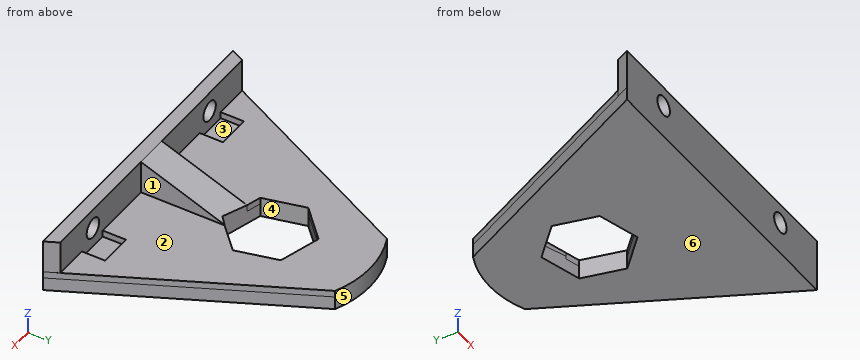
```python
from build123d import *

# Parameters (mm, degrees)
SKETCH_1_R               = 3
EXTRUDE_1_DEPTH          = 2
EXTRUDE_2_DEPTH          = 6
RIB_2_REACH              = 42.702
SKETCH_3_WALL_W          = 109.004825052
SKETCH_3_WALL_H          = 5
SKETCH_4_R               = 4.101413307
EXTRUDE_3_DEPTH          = 2
EXTRUDE_START            = -3
EXTRUDE_4_DEPTH          = 1
CUT_EXTRUDE_1_DEPTH      = 41.220101475
CUT_EXTRUDE_1_DEPTH_BACK = 41.220101475
CUT_EXTRUDE_2_DEPTH      = 10
CUT_EXTRUDE_3_DEPTH      = 10
SKETCH_14_R              = 1.5
CUT_EXTRUDE_4_DEPTH      = 10
SKETCH_15_W              = 5.01110436
SKETCH_15_H              = 3.494287521
CUT_EXTRUDE_5_DEPTH      = 1


# Read off the part's stored shape, not the designer's step: the extrude step
with BuildPart() as part:
    # Sketch 1 → Extrude 1 (new body)
    with BuildSketch(Plane.XY):
        with BuildLine():
            Line((-5.382175267, 2.651827558), (-22.819924686, -32.74))
            Line((-22.819924686, -32.74), (22.819924686, -32.74))
            Line((22.819924686, -32.74), (5.382175267, 2.651827558))
            ThreePointArc((5.382175267, 2.651827558), (0, 6), (-5.382175267, 2.651827558))
        make_face()
        Circle(SKETCH_1_R, mode=Mode.SUBTRACT)
    extrude(amount=EXTRUDE_1_DEPTH)

    # Sketch 2 → Extrude 2 (add)
    with BuildSketch(Plane.XY.offset(2)):
        Polygon((21.824193002, -30.74), (22.819924686, -32.74), (-22.819924686, -32.74), (-21.851665672, -30.74), align=None)
    extrude(amount=EXTRUDE_2_DEPTH)

    # Sketch 3 wall → Rib 2 (add, up to next)
    with BuildSketch(Plane(origin=(0, -18.296150966, 5), x_dir=(0, -0.972147881588, 0.234368292061), z_dir=(0, -0.234368292061, -0.972147881588)), mode=Mode.PRIVATE) as rib_2_sk1:
        Rectangle(SKETCH_3_WALL_W, SKETCH_3_WALL_H)
    rib_2_tool1 = extrude(rib_2_sk1.sketch, amount=RIB_2_REACH, mode=Mode.PRIVATE) - part.part
    add(rib_2_tool1.solids().sort_by_distance((0, -18.296150966, 5))[0])

    # Sketch 4 → Extrude 3 (add)
    with BuildSketch(Plane.XY.offset(2)):
        Circle(SKETCH_4_R)
    extrude(amount=-EXTRUDE_3_DEPTH)

    # Extrude 4 outline → Extrude 4 (add)
    with BuildSketch(Plane(origin=(0, 0, 0), x_dir=(-1, 0, 0), z_dir=(0, 0, -1)).offset(EXTRUDE_START)):
        with BuildLine():
            Line((-6.23517922, 0.920562354), (-22.819924686, -32.74))
            Line((-22.819924686, -32.74), (-21.824193002, -30.74))
            Line((-21.824193002, -30.74), (-2.5, -30.74))
            Line((-2.5, -30.74), (-2.5, -18.104077215))
            Line((-2.5, -18.104077215), (-6.21139304, -14.53775689))
            Line((-6.21139304, -14.53775689), (-4.662599656, -8.259654279))
            Line((-4.662599656, -8.259654279), (-2.5, -7.633735358))
            Line((-2.5, -7.633735358), (1.548793384, -6.461897389))
            Line((1.548793384, -6.461897389), (2.5, -7.375922784))
            Line((2.5, -7.375922784), (6.21139304, -10.94224311))
            Line((6.21139304, -10.94224311), (4.662599656, -17.220345721))
            Line((4.662599656, -17.220345721), (2.5, -17.846264642))
            Line((2.5, -17.846264642), (2.5, -30.74))
            Line((2.5, -30.74), (21.834513611, -30.74))
            Line((21.834513611, -30.74), (6.23517922, 0.920562354))
            ThreePointArc((6.23517922, 0.920562354), (0, 2.276271965), (-6.23517922, 0.920562354))
        make_face()
    extrude(amount=EXTRUDE_4_DEPTH)

    # Sketch 11 → Cut-Extrude 1 (cut, two sides: drawn at the far end of the back side and taken through both)
    with BuildSketch(Plane.XY.offset(3).offset(-CUT_EXTRUDE_1_DEPTH_BACK)):
        Polygon((6.21139304, -14.53775689), (4.662599656, -8.259654279), (-1.548793384, -6.461897389), (-6.21139304, -10.94224311), (-4.662599656, -17.220345721), (1.548793384, -19.018102611), align=None)
    extrude(amount=CUT_EXTRUDE_1_DEPTH + CUT_EXTRUDE_1_DEPTH_BACK, mode=Mode.SUBTRACT)

    # Sketch 12 → Cut-Extrude 2 (cut)
    with BuildSketch(Plane.XY.offset(3)):
        with BuildLine():
            Line((14.504971028, 2.702486536), (10.280667783, -1.794850678))
            ThreePointArc((10.280667783, -1.794850678), (0.290112641, 2.273469232), (-9.850153994, -1.405852921))
            Line((-9.850153994, -1.405852921), (-13.409584794, 3.662670837))
            ThreePointArc((-13.409584794, 3.662670837), (0.728324257, 8.43390183), (14.504971028, 2.702486536))
        make_face()
    extrude(amount=-CUT_EXTRUDE_2_DEPTH, mode=Mode.SUBTRACT)

    # Sketch 13 → Cut-Extrude 3 (cut)
    with BuildSketch(Plane.ZY.offset(2.5)):
        Polygon((3, -17.846264642), (8, -30.74), (8, -17.846264642), (3.4065387, -17.846264642), align=None)
    extrude(amount=-CUT_EXTRUDE_3_DEPTH, mode=Mode.SUBTRACT)

    # Sketch 14 → Cut-Extrude 4 (cut)
    with BuildSketch(Plane.XZ.offset(32.74)):
        with Locations(Location((14.013848445, 5.011131475, 0), (0, 0, 270))):
            Circle(SKETCH_14_R)
        with Locations(Location((-14.013847957, 5.011131475, 0), (0, 0, 270))):
            Circle(SKETCH_14_R)
    extrude(amount=-CUT_EXTRUDE_4_DEPTH, mode=Mode.SUBTRACT)

    # Sketch 15 → Cut-Extrude 5 (cut)
    with BuildSketch(Plane.XY.offset(3)):
        with Locations((-14.168501734, -28.99285624)):
            Rectangle(SKETCH_15_W, SKETCH_15_H)
        with Locations((14.168501734, -28.99285624)):
            Rectangle(SKETCH_15_W, SKETCH_15_H)
    extrude(amount=-CUT_EXTRUDE_5_DEPTH, mode=Mode.SUBTRACT)


solid = part.part
```
Work out the finished part from the listing and answer in its coordinate system (mm). Face numbers are marked on the shaded views. A direction names the side the tool comes from. Coordinates: 2 decimals unless noted, no trailing zeros. Write each loop counter-clockwise with the first axis right and the second up, starting at its lowest first coordinate (ties: lowest second). Pieces come first, ordered by that corner, then holes. Notation, with made-up numbers: (88, -32.5) - (124, -32.5) arc R32 ccw to (124, 4.5) - close; hole circle Ø7 at (13.25, -19). An arc over 180 degrees is marked (long way). Answer as a JSON object with one key per item and string values.
Q1. Find section C-C (x = 16). Write down the section's boundary in (y, z), plus the area to 3 significant figures.
Results list:
{"outline": "(-32.74, 0) - (-18.9, 0) - (-18.9, 3) - (-27.25, 3) - (-27.25, 2) - (-30.74, 2) - (-30.74, 8) - (-32.74, 8) - close", "area": "48.0 mm^2"}
Q2. Consider L1, parallel to Z at x = 9, y = -21; L2, parallel to X at y = -27, z = 4; L3, parallel to Y at x = 9.5, z = 3.5. Determine where each line is inside the solid, lowest interval first. Write a range as from..to.
Results list:
{"L1": "z = 0..3", "L2": "x = -2.5..2.5", "L3": "y = -32.74..-30.74"}
Q3. Find section A-A (y = -10). Write down the section's boundary in (x, z).
Results list:
{"outline": "(-11.62, 0) - (-5.23, 0) - (-5.23, 3) - (-11.62, 3) - close; (5.09, 0) - (11.62, 0) - (11.62, 3) - (5.09, 3) - close"}
Q4. Find section D-D (y = -25). Write down the section's boundary in (x, z).
Results list:
{"outline": "(-19.01, 0) - (19.01, 0) - (19.01, 3) - (2.5, 3) - (2.5, 5.77) - (-2.5, 5.77) - (-2.5, 3) - (-19.01, 3) - close"}
Q5. For a pull along Y with two mould halves and no side action, classify the marked faces 4, 5 and 6 as pulls with the +Y half, pulls with the -Y half, needs draft (parallel to the pull), parting line crosses it, or undercut.
Results list:
{"face 4": "undercut", "face 5": "pulls with the +Y half", "face 6": "needs draft"}
Q6. Given pin 1 Ø1.1 at (y, z) = (-28, 2.5) entering from +X; pin 2 Ø2 at (y, z) = (-15.5, 2.5) entering from -X; pin 3 Ø3 at (x, z) = (-14, 5.5) entering from +Y; pin 4 Ø4 at (y, z) = (-18, 6.5) entering from -X, each flat-ended and moving along its own axis, determine where each tip first touches the part or whether it passes through.
Results list:
{"pin 1": "stops at x = 20.76", "pin 2": "stops at x = -14.82", "pin 3": "stops at y = -30.74", "pin 4": "passes through"}
Q7. Which of the six approach directions +Z, -Z, +X, -X, +Y, -Y give full straight-line access (tool end or side, diameter ignored) to the marked faces 1, 2 and 3?
Results list:
{"face 1": "+Z, +X, +Y", "face 2": "+Z, +Y", "face 3": "+Z"}
Q8. Find section B-B (z = 4.75). Write down the section's boundary in (x, y), plus the area to 3 significant figures.
Results list:
{"outline": "(-22.82, -32.74) - (-15.49, -32.74) - (-15.49, -30.74) - (-21.85, -30.74) - close; (-12.54, -32.74) - (12.54, -32.74) - (12.54, -30.74) - (2.5, -30.74) - (2.5, -22.36) - (-2.5, -22.36) - (-2.5, -30.74) - (-12.54, -30.74) - close; (15.49, -32.74) - (22.82, -32.74) - (21.82, -30.74) - (15.49, -30.74) - close", "area": "119 mm^2"}
